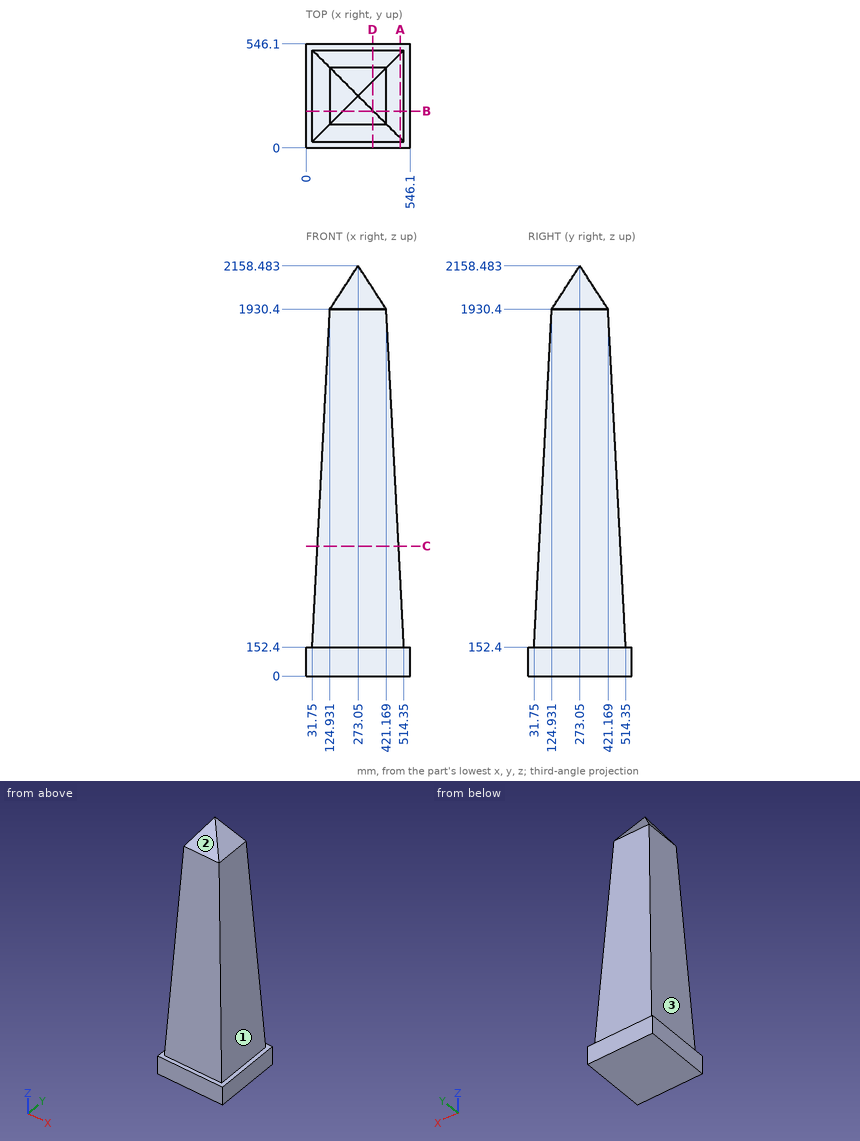
The figure shows three views and two pictorial views of one solid part (mm, origin at its lowest corner). Answer the questions. Give positions to 0.01 mm unless a question says otherwise; leave off trailing zeros. Write each loop counter-clockwise with the first axis right and the second up, starting at its lowest first coordinate (ties: lowest second). Pieces come first, ordered by that corner, then holes. Notation, with made-up numbers: (67, 33) - (91, 33) arc R15 ccw to (91, 45) - close; hole circle Ø2 at (-25.5, 12.25). An arc over 180 degrees is marked (long way). Use CSV: the item, a comma, the result in double quotes. Start each with the question number.
Item 1: The part is cut by section B-B, the plane y = 192.5. Give the vertices of the cut face in (x, z), and give its area (3 significant figures).
Item 2: The part is cut by section C-C, the plane z = 683. Give the vertices of the cut face in (x, y), and give its area (3 significant figures).
Item 3: Consider line 1 (X direction, y = 386.5, z = 198.5); line 2 (Y direction, x = 344, z = 513); line 3 (Y direction, x = 390, z = 1382). Determine where each line is inside the solid, lowest interval first.
Item 4: The part is cut by section A-A, the plane x = 495. Give the vertices of the cut face in (y, z).
Item 5: Flat-ended cylindrical pins translate along their axes: P1, Ø10, axis at x = 356.5, y = 314, coming from the +Z side; P2, Ø5, axis at x = 298, z = 1071.5, coming from the -Y side; P3, Ø5, axis at x = 405.5, y = 323, coming from the +Z side; P4, Ø10, axis at x = 371.5, y = 70.5, coming from the -Z side. Find the tip coordinate at first contact, or state that the pin passes through.
Item 6: The mould has two halves that part along X. Classify the marked faces 1, 2 and 3: pulls with the +X half, pulls with the -X half, needs draft (parallel to the pull), parting line crosses it, or undercut.
Item 7: The part is cut by section D-D, the plane x = 349.5. Give the vertices of the cut face in (y, z).
Taken from the geometry:
1,outline,"(0, 0) - (546.1, 0) - (546.1, 152.4) - (514.35, 152.4) - (421.17, 1930.4) - (353.6, 2034.45) - (192.5, 2034.45) - (124.93, 1930.4) - (31.75, 152.4) - (0, 152.4) - close"
1,area,"799,000 mm2"
2,outline,"(59.56, 59.56) - (486.54, 59.56) - (486.54, 486.54) - (59.56, 486.54) - close"
2,area,"182,000 mm2"
3,line 1,"34.17 to 511.93"
3,line 2,"50.65 to 495.45"
3,line 3,"96.19 to 449.91"
4,outline,"(0, 0) - (546.1, 0) - (546.1, 152.4) - (514.35, 152.4) - (495, 521.62) - (51.1, 521.62) - (31.75, 152.4) - (0, 152.4) - close"
5,P1,"z = 2037.68"
5,P2,"y = 79.79"
5,P3,"z = 1958.38"
5,P4,"z = 0"
6,face 1,"pulls with the +X half"
6,face 2,"needs draft"
6,face 3,"pulls with the -X half"
7,outline,"(0, 0) - (546.1, 0) - (546.1, 152.4) - (514.35, 152.4) - (421.17, 1930.4) - (349.5, 2040.76) - (196.6, 2040.76) - (124.93, 1930.4) - (31.75, 152.4) - (0, 152.4) - close"
